Read the model definition and answer for the solid it produces. Units are mm, in the model's axes. A direction names the side the tool comes from. Give positions to 0.01 mm unless a question says otherwise; leave off trailing zeros. Loops run counter-clockwise (first coordinate to the right, second up) from the corner with the lowest first, then second, coordinate; pieces in that order, holes last. Notation, with made-up numbers: (45.25, 2.5) - (90.25, 2.5) arc R12 cw to (90.25, 25.5) - close; hole circle Ø11 at (68.5, 19). An arc over 180 degrees is marked (long way). Put each result on its own line as item: value. Start each with the question number.
1. A cutting plane is placed at B-B, the plane z = -13.5. Count the separate pieces of the cut face and the enclosed holes in it, plus the area to 3 significant figures.
2. For a pull along Y with two mould halves and no side action, classify faces 1 (the cylindrical face through (-220.49, -45.72, -12.68)), 2 (the cylindrical face through (-218.39, 63.58, -2.46)), 3 (the flat face through (3, 70, -12)) as released by +Y, released by -Y, zero draft, split by the parting line, or undercut.
3. A cutting plane is placed at D-D, the plane x = -165. Determine the outline of the cut face in (y, z).
4. Consider L1, parallel to Y at x = 0, z = -8; L2, parallel to Y at x = -118, z = -3; L3, parallel to Y at x = 55, z = -18. Determine where each line is inside the solid, lowest interval first. Write a range as from..to.
5. A cutting plane is placed at C-C, the plane y = 25. Determine the outline of the cut face in (x, z).
6. A cutting plane is placed at A-A, the plane x = -55. Determine the outline of the cut face in (y, z).
7. Given pin 1 Ø6 at (x, y) = (-123.5, -51.5) entering from -Z; pin 2 Ø9.5 at (x, y) = (0, -25) entering from +Z; pin 3 Ø2 at (x, z) = (-174, -9.5) entering from -Y; pin 4 Ø1.8 at (x, y) = (99, 43.5) entering from +Z, each flat-ended and moving along its own axis, determine where each tip first touches the part or whether it passes through.
8. For faces 4 (the cylindrical face through (220.49, -65.72, -12.68)), 5 (the cylindrical face through (218.39, -63.58, -2.46)), determine the directions among +Z, -Z, +X, -X, +Y, -Y from which every point of the face is accessible in a straight line to the end or side of a thin tool.
```python
from build123d import *

# Parameters (mm, degrees)
BOSS_EXTRUDE1_DEPTH = 25
FILLET1_R           = 15
SKETCH2_R           = 50
SKETCH2_R_2         = 22.5
SKETCH2_R_3         = 7.5
CUT_EXTRUDE1_DEPTH  = 237.959912221
CUT_EXTRUDE2_DEPTH  = 5
SKETCH5_R           = 3
CUT_EXTRUDE3_DEPTH  = 12.7


with BuildPart() as part:
    # Sketch1 → Boss-Extrude1 (new body)
    with BuildSketch(Plane.XY):
        Polygon((-225, -50), (-110, -50), (-93.218007376, -70), (225, -70), (225, 70), (-225, 70), align=None)
    extrude(amount=-BOSS_EXTRUDE1_DEPTH)

    # Fillet1
    fillet1_edges = [part.edges().sort_by_distance(p)[0] for p in [
        (225, -70, -12.5),
        (-93.218007376, -70, -12.5),
        (-110, -50, -12.5),
        (-225, -50, -12.5),
        (-225, 70, -12.5),
        (225, 70, -12.5),
    ]]
    fillet(fillet1_edges, radius=FILLET1_R)

    # Sketch2 → Cut-Extrude1 (cut, through all)
    with BuildSketch(Plane.XY):
        with Locations((55, 0)):
            Circle(SKETCH2_R)
        with Locations((127, 25)):
            Circle(SKETCH2_R_2)
        with Locations((165, -20)):
            Circle(SKETCH2_R_2)
        with Locations(Location((-165, -20, 0), (0, 0, 180))):
            Circle(SKETCH2_R_2)
        with Locations(Location((-127, 25, 0), (0, 0, 180))):
            Circle(SKETCH2_R_2)
        with Locations(Location((-55, 0, 0), (0, 0, 180))):
            Circle(SKETCH2_R)
        with Locations((-115, -15)):
            Circle(SKETCH2_R_3)
    extrude(amount=-CUT_EXTRUDE1_DEPTH, mode=Mode.SUBTRACT)

    # Sketch4 → Cut-Extrude2 (cut)
    with BuildSketch(Plane.XY):
        with BuildLine():
            Line((-103.205814896, -53.429823026), (-95.415925822, -62.713451316))
            ThreePointArc((-95.415925822, -62.713451316), (-91.294811645, -65.875693444), (-86.223392504, -67))
            Line((-86.223392504, -67), (210, -67))
            ThreePointArc((210, -67), (218.485281374, -63.485281374), (222, -55))
            Line((222, -55), (222, 55))
            ThreePointArc((222, 55), (218.485281374, 63.485281374), (210, 67))
            Line((210, 67), (-210, 67))
            ThreePointArc((-210, 67), (-218.485281374, 63.485281374), (-222, 55))
            Line((-222, 55), (-222, -35))
            ThreePointArc((-222, -35), (-218.485281374, -43.485281374), (-210, -47))
            Line((-210, -47), (-116.994614872, -47))
            ThreePointArc((-116.994614872, -47), (-109.387486161, -48.686459833), (-103.205814896, -53.429823026))
        make_face()
    extrude(amount=-CUT_EXTRUDE2_DEPTH, mode=Mode.SUBTRACT)

    # Sketch5 → Cut-Extrude3 (cut)
    with BuildSketch(Plane.XY.offset(-5)):
        with Locations((0, 45)):
            Circle(SKETCH5_R)
        with Locations((0, -25)):
            Circle(SKETCH5_R)
        with Locations((100, 45)):
            Circle(SKETCH5_R)
        with Locations((-96.85, 45)):
            Circle(SKETCH5_R)
    extrude(amount=-CUT_EXTRUDE3_DEPTH, mode=Mode.SUBTRACT)


solid = part.part
```
Return value:
1. separate pieces: 1
1. enclosed holes: 11
1. area: 38,000 mm2
2. face 1: released by -Y
2. face 2: undercut
2. face 3: released by +Y
3. outline: (-50, -25) - (-42.5, -25) - (-42.5, -5) - (-47, -5) - (-47, 0) - (-50, 0) - close; (2.5, -25) - (70, -25) - (70, 0) - (67, 0) - (67, -5) - (2.5, -5) - close
4. L1: y = -70..-28, -22..42, 48..70
4. L2: y = -50..-47, 67..70
4. L3: y = -70..-50, 50..70
5. outline: (-225, -25) - (-149.5, -25) - (-149.5, -5) - (-222, -5) - (-222, 0) - (-225, 0) - close; (-104.5, -25) - (-98.3, -25) - (-98.3, -5) - (-104.5, -5) - close; (-11.7, -25) - (11.7, -25) - (11.7, -5) - (-11.7, -5) - close; (98.3, -25) - (104.5, -25) - (104.5, -5) - (98.3, -5) - close; (149.5, -25) - (225, -25) - (225, 0) - (222, 0) - (222, -5) - (149.5, -5) - close
6. outline: (-70, -25) - (-50, -25) - (-50, -5) - (-67, -5) - (-67, 0) - (-70, 0) - close; (50, -25) - (70, -25) - (70, 0) - (67, 0) - (67, -5) - (50, -5) - close
7. pin 1: stops at z = -25
7. pin 2: stops at z = -5
7. pin 3: stops at y = -50
7. pin 4: stops at z = -17.7
8. face 4: +Z, -Z, +X, -Y
8. face 5: +Z
